from build123d import *

# Parameters (mm, degrees)
EXTRUDE_THIN1_DEPTH = 25


with BuildPart() as part:
    # Sketch3 → Extrude-Thin1 (new body, symmetric)
    with BuildSketch(Plane(origin=(0, 0, 0), x_dir=(0, 0, -1), z_dir=(1, 0, 0))):
        Polygon((0, 4.75), (10.175645864, 4.75), (11.801837516, 9.26259239), (15.405512547, -0.73740761), (19.009187578, 9.26259239), (22.612862609, -0.73740761), (26.21653764, 9.26259239), (29.820212671, -0.73740761), (33.423887702, 9.26259239), (37.027562733, -0.73740761), (40.631237764, 9.26259239), (44.234912795, -0.73740761), (47.838587827, 9.26259239), (51.442262858, -0.73740761), (55.045937889, 9.26259239), (58.64961292, -0.73740761), (62.253287951, 9.26259239), (65.856962982, -0.73740761), (69.460638013, 9.26259239), (73.064313044, -0.73740761), (76.667988075, 9.26259239), (80.271663106, -0.73740761), (83.875338138, 9.26259239), (87.479013169, -0.73740761), (91.0826882, 9.26259239), (94.686363231, -0.73740761), (98.290038262, 9.26259239), (99.916229914, 4.75), (110.091875777, 4.75), (110.091875777, 5.25), (100.267521641, 5.25), (98.290038262, 10.73740761), (94.686363231, 0.73740761), (91.0826882, 10.73740761), (87.479013169, 0.73740761), (83.875338138, 10.73740761), (80.271663106, 0.73740761), (76.667988075, 10.73740761), (73.064313044, 0.73740761), (69.460638013, 10.73740761), (65.856962982, 0.73740761), (62.253287951, 10.73740761), (58.64961292, 0.73740761), (55.045937889, 10.73740761), (51.442262858, 0.73740761), (47.838587827, 10.73740761), (44.234912795, 0.73740761), (40.631237764, 10.73740761), (37.027562733, 0.73740761), (33.423887702, 10.73740761), (29.820212671, 0.73740761), (26.21653764, 10.73740761), (22.612862609, 0.73740761), (19.009187578, 10.73740761), (15.405512547, 0.73740761), (11.801837516, 10.73740761), (9.824354136, 5.25), (0, 5.25), align=None)
    extrude(amount=EXTRUDE_THIN1_DEPTH, both=True)


solid = part.part
Verification items for the finished model (mm, model axes). A direction names the side the tool comes from. Give positions to 0.01 mm unless a question says otherwise; leave off trailing zeros. Loops run counter-clockwise (first coordinate to the right, second up) from the corner with the lowest first, then second, coordinate; pieces in that order, holes last.
1) Draft check along Z on faces 1 (the flat face through (0, 4.75, -5)), 2 (the flat face through (0.35, 4.193, -89.256)), 3 (the flat face through (0.35, 7.96, -99.29)). Enter one of: pulls with the +Z half, pulls with the -Z half, needs draft (parallel to the pull), parting line crosses it, or undercut.
2) Depth check by flat-ended pin: pin 1 Ø8 at (x, z) = (11.5, -60) entering from +Y; pin 2 Ø3 at (x, z) = (12, -107.5) entering from +Y; pin 3 Ø5 at (x, y) = (-17.5, 1) entering from -Z. Enter the tip coordinate at first touch or a pass-through.
3) Thickness scan on line 1 along Y through (x, z) = (-21.5, -5). Record the ranges inside material, lowest first.
4) Sectioned sample at A-A, the plane y = 7.75. Count the separate pieces of the cut face and the enclosed holes in it, then the cut area to 3 significant figures.
5) Set-up check for faces 4 (the flat face through (0.35, 5.807, -89.306)), 5 (the flat face through (0.35, 4.193, -67.634)), 6 (the flat face through (25, 9.3, -54.8)): record each of +Z, -Z, +X, -X, +Y, -Y from which the full face is reachable in a straight line by a thin tool's end or side.
6) Sectioned sample at D-D, the plane z = -57. Enter the section's corners in (x, y) (3 decimals), then the cut area to 3 significant figures.
7) Sectioned sample at B-B, the plane z = -8. Enter the section's corners in (x, y), then the cut area to 3 significant figures.
Answers:
1. face 1: needs draft
1. face 2: undercut
1. face 3: pulls with the -Z half
2. pin 1: stops at y = 10.74
2. pin 2: stops at y = 5.25
2. pin 3: stops at z = -96.21
3. line 1: y = 4.75 to 5.25
4. separate pieces: 26
4. enclosed holes: 0
4. area: 691 mm2
5. face 4: +X, -X, +Y
5. face 5: +X, -X, -Y
5. face 6: +Z, -Z, +X, +Y, -Y
6. outline: (-25, 3.84) - (25, 3.84) - (25, 5.315) - (-25, 5.315) - close
6. area: 73.7 mm2
7. outline: (-25, 4.75) - (25, 4.75) - (25, 5.25) - (-25, 5.25) - close
7. area: 25.0 mm2
